The listing builds one solid part. Answer for the finished solid, in the listing's coordinates (mm). A direction names the side the tool comes from. Coordinates: 2 decimals unless noted, no trailing zeros. Write each loop counter-clockwise with the first axis right and the second up, starting at its lowest first coordinate (ties: lowest second). Pieces come first, ordered by that corner, then holes.
```python
from build123d import *

# Parameters (mm, degrees)
SKETCH1_W                        = 254
SKETCH1_H                        = 76.2
BOSS_EXTRUDE1_DEPTH              = 25.4
SHELL1_T                         = -3.175
SKETCH2_R                        = 14.2875
SKETCH2_R_2                      = 2.4892
CUT_EXTRUDE1_DEPTH               = 136.002851822
F_10_CLEARANCE_HOLE1_D           = 4.9784
F_3_8_0_375_DIAMETER_HOLE1_D     = 9.525
F_3_8_0_375_DIAMETER_HOLE1_DEPTH = 10.922
F_3_8_0_375_DIAMETER_HOLE1_TIP   = 2.861598698
F_3_8_0_375_DIAMETER_HOLE2_D     = 9.525
F_3_8_0_375_DIAMETER_HOLE2_DEPTH = 10.922
F_3_8_0_375_DIAMETER_HOLE2_TIP   = 2.861598698
SKETCH11_R                       = 2.4892
CUT_EXTRUDE2_DEPTH               = 151.268426491


with BuildPart() as part:
    # Sketch1 → Boss-Extrude1 (new body)
    with BuildSketch(Plane(origin=(0, 0, 0), x_dir=(0, 0, -1), z_dir=(1, 0, 0))):
        Rectangle(SKETCH1_W, SKETCH1_H)
    extrude(amount=BOSS_EXTRUDE1_DEPTH)

    # Shell1
    shell1_openings = [part.faces().sort_by_distance(p)[0] for p in [
        (12.7, 0, 127),
        (12.7, 0, -127),
    ]]
    offset(amount=SHELL1_T, openings=shell1_openings, kind=Kind.INTERSECTION)

    # Sketch2 → Cut-Extrude1 (cut, through all)
    with BuildSketch(Plane(origin=(25.4, 0, 0), x_dir=(0, 0, -1), z_dir=(1, 0, 0))):
        with Locations((0, -6.35)):
            Circle(SKETCH2_R)
        with Locations((-82.55, -6.35)):
            Circle(SKETCH2_R)
        with Locations((82.55, -6.35)):
            Circle(SKETCH2_R)
        with Locations((-41.275, 16.51)):
            Circle(SKETCH2_R_2)
        with Locations((-41.275, -27.94)):
            Circle(SKETCH2_R_2)
        with Locations((41.275, -27.94)):
            Circle(SKETCH2_R_2)
        with Locations((41.275, 16.51)):
            Circle(SKETCH2_R_2)
        with Locations((-54.61, 27.94)):
            Circle(SKETCH2_R_2)
        with Locations((-54.61, -13.97)):
            Circle(SKETCH2_R_2)
        with Locations((41.91, -13.97)):
            Circle(SKETCH2_R_2)
        with Locations((41.91, 27.94)):
            Circle(SKETCH2_R_2)
    extrude(amount=-CUT_EXTRUDE1_DEPTH, mode=Mode.SUBTRACT)

    # #10 Clearance Hole1 (through all)
    with Locations(Plane(origin=(25.4, 0, 0), x_dir=(0, 0, -1), z_dir=(1, 0, 0))):
        with Locations((-120.904, 19.05), (-120.904, -19.05)):
            f_10_clearance_hole1 = Hole(F_10_CLEARANCE_HOLE1_D / 2)

    # Mirror1: #10 Clearance Hole1 across plane
    add(f_10_clearance_hole1.mirror(Plane.XY), mode=Mode.SUBTRACT)

    # 3/8 (0.375) Diameter Hole1
    with Locations(Plane.ZY):
        with Locations((54.61, 27.94), (54.61, -13.97), (-41.91, -13.97), (-41.91, 27.94)):
            Hole(F_3_8_0_375_DIAMETER_HOLE1_D / 2, depth=F_3_8_0_375_DIAMETER_HOLE1_DEPTH)
            with Locations((0, 0, -(F_3_8_0_375_DIAMETER_HOLE1_DEPTH + F_3_8_0_375_DIAMETER_HOLE1_TIP / 2))):  # 118° drill point
                Cone(0, F_3_8_0_375_DIAMETER_HOLE1_D / 2, F_3_8_0_375_DIAMETER_HOLE1_TIP, mode=Mode.SUBTRACT)

    # 3/8 (0.375) Diameter Hole2
    with Locations(Plane(origin=(25.4, 0, 0), x_dir=(0, 0, -1), z_dir=(1, 0, 0))):
        with Locations((-41.275, 16.51), (-41.275, -27.94), (41.275, 16.51), (41.275, -27.94)):
            Hole(F_3_8_0_375_DIAMETER_HOLE2_D / 2, depth=F_3_8_0_375_DIAMETER_HOLE2_DEPTH)
            with Locations((0, 0, -(F_3_8_0_375_DIAMETER_HOLE2_DEPTH + F_3_8_0_375_DIAMETER_HOLE2_TIP / 2))):  # 118° drill point
                Cone(0, F_3_8_0_375_DIAMETER_HOLE2_D / 2, F_3_8_0_375_DIAMETER_HOLE2_TIP, mode=Mode.SUBTRACT)

    # Sketch11 → Cut-Extrude2 (cut, through all)
    with BuildSketch(Plane.XZ.offset(38.1)):
        with Locations(Location((12.7, -110.49, 0), (0, 0, 270))):
            Circle(SKETCH11_R)
        with Locations(Location((12.7, -66.294, 0), (0, 0, 270))):
            Circle(SKETCH11_R)
        with Locations(Location((12.7, -22.098, 0), (0, 0, 270))):
            Circle(SKETCH11_R)
        with Locations(Location((12.7, 22.098, 0), (0, 0, 270))):
            Circle(SKETCH11_R)
        with Locations(Location((12.7, 66.294, 0), (0, 0, 270))):
            Circle(SKETCH11_R)
        with Locations(Location((12.7, 110.49, 0), (0, 0, 270))):
            Circle(SKETCH11_R)
    extrude(amount=-CUT_EXTRUDE2_DEPTH, mode=Mode.SUBTRACT)


solid = part.part
```
(1) For a pull along Z with two mould halves and no side action, classify faces 1 (the flat face through (13, 34.925, 2)), 2 (the cylindrical face through (1.61, 14.08, -40.74)) as pulls with the +Z half, pulls with the -Z half, needs draft (parallel to the pull), parting line crosses it, or undercut.
(2) Section D-D, the plane y = 27.94 is taken. Write down the section's boundary in (x, z) (1 decimal), plus the area to 3 significant figures.
(3) Section B-B, the plane y = -6.35 is taken. State how many separate pieces and enclosed holes the cut face has, plus the area to 3 significant figures.
(4) Section C-C, the plane x = 18.25 is taken. Write down the section's boundary in (y, z) (3 decimals), plus the area to 3 significant figures.
(5) Which of the six approach directions +Z, -Z, +X, -X, +Y, -Y give full straight-line access (tool end or side, diameter ignored) to faces 3 (the flat face through (13, -34.925, 2)), 4 (the cylindrical face through (23.79, 13.612, 37.496)), 5 (the cylindrical face through (1.61, 28.149, -37.152))?
(6) This flat-tipped pin is pushed along its axis until it touches: pin 1 (8 mm diameter, centred on y = -19.05, z = 120.904, fed in from -X). Where does it stop, or does it pass through?
(7) Section A-A, the plane z = 82.55 is taken. Write down the section's boundary in (x, y) (1 decimal).
(8) Find the intervals of material crossed by probe 1 along X at (y, z) = (-32, 19.5) (3 decimals); probe 2 along Y at (x, z) = (4, 32) (3 decimals); probe 3 along Y at (x, z) = (24.45, -82.55), in increasing order.
Solution:
1. face 1: needs draft
1. face 2: undercut
2. outline: (0, -127) - (3.2, -127) - (3.2, -46.7) - (0, -46.7) - close; (0, -37.1) - (3.2, -37.1) - (3.2, 49.8) - (0, 49.8) - close; (0, 59.4) - (3.2, 59.4) - (3.2, 127) - (0, 127) - close; (22.2, -127) - (25.4, -127) - (25.4, -44.4) - (22.2, -44.4) - close; (22.2, -39.4) - (25.4, -39.4) - (25.4, 52.1) - (22.2, 52.1) - close; (22.2, 57.1) - (25.4, 57.1) - (25.4, 127) - (22.2, 127) - close
2. area: 1,520 mm2
3. separate pieces: 8
3. enclosed holes: 0
3. area: 1,070 mm2
4. outline: (-38.1, -127) - (-34.925, -127) - (-34.925, 127) - (-38.1, 127) - close; (34.925, -127) - (38.1, -127) - (38.1, 127) - (34.925, 127) - close
4. area: 1,610 mm2
5. face 3: +Z, -Z
5. face 4: +X
5. face 5: -X
6. pin 1: stops at x = 0
7. outline: (0, -38.1) - (25.4, -38.1) - (25.4, -20.6) - (22.2, -20.6) - (22.2, -34.9) - (3.2, -34.9) - (3.2, -20.6) - (0, -20.6) - close; (0, 7.9) - (3.2, 7.9) - (3.2, 34.9) - (22.2, 34.9) - (22.2, 7.9) - (25.4, 7.9) - (25.4, 38.1) - (0, 38.1) - close
8. probe 1: x = 0 to 3.175, 22.225 to 25.4
8. probe 2: y = -38.1 to -34.925, 34.925 to 38.1
8. probe 3: y = -38.1 to -20.64, 7.94 to 38.1
